Geometry check sheet. Reference: the model listing, model coordinates, mm. Coordinates: 2 decimals unless noted, no trailing zeros. Loops run counter-clockwise (first coordinate to the right, second up) from the corner with the lowest first, then second, coordinate; pieces in that order, holes last.
from build123d import *

# Parameters (mm, degrees)
SKETCH_1_R      = 6
SKETCH_1_R_2    = 3.3
EXTRUDE_1_DEPTH = 5


with BuildPart() as part:
    # 스케치1 → 보스-돌출1 (new body)
    with BuildSketch(Plane(origin=(0, 0, 0), x_dir=(1, 0, 0), z_dir=(0, 1, 0))):
        Circle(SKETCH_1_R)
        Circle(SKETCH_1_R_2, mode=Mode.SUBTRACT)
        with BuildLine():
            Line((-5.795554958, -1.552914271), (-1.448888739, -17.774893441))
            ThreePointArc((-1.448888739, -17.774893441), (0, -18.886664873), (1.448888739, -17.774893441))
            Line((1.448888739, -17.774893441), (5.795554958, -1.552914271))
            ThreePointArc((5.795554958, -1.552914271), (0, -6), (-5.795554958, -1.552914271))
        make_face()
    extrude(amount=EXTRUDE_1_DEPTH)


solid = part.part
1) Section check D-D on x = -4.25. Record the cut outline in (y, z).
Data:
outline: (0, -4.24) - (5, -4.24) - (5, 7.32) - (0, 7.32) - close
2) Mould release check, pull along Z, two halves, no side actions. Record for faces 1 (the flat face through (-3.653, 2.465, 9.55)), 2 (the flat face through (0, 0, 6)), 3 (the cylindrical face through (0, 2, -6)), 4 (the cylindrical face through (-2.43, 2.46, -2.23)): +Z half, -Z half, draft (parallel to the pull), parting line (faces both ways), or undercut.
Data:
face 1: +Z half
face 2: draft
face 3: parting line
face 4: undercut
3) Depth check by flat-ended pin: pin 1 (1.5 mm diameter, centred on y = 2.5, z = 11.5, fed in from +X); pin 2 (1 mm diameter, centred on y = 2, z = 14.5, fed in from +X); pin 3 (2 mm diameter, centred on y = 3, z = 3, fed in from +X); pin 4 (3 mm diameter, centred on x = 2.5, z = 15, fed in from -Y). Enter the tip coordinate at first touch or a pass-through.
Data:
pin 1: stops at x = 3.33
pin 2: stops at x = 2.46
pin 3: stops at x = 5.68
pin 4: stops at y = 0
4) Section check C-C on y = 3.2. Record the cut outline in (x, z), and give its area (3 significant figures).
Data:
outline: (-5.8, 1.55) arc R6 ccw (long way) to (5.8, 1.55) - (1.45, 17.77) arc R1.5 ccw to (-1.45, 17.77) - close; hole circle Ø6.6 at (0, 0)
area: 161 mm2
5) Section check A-A on z = 0. Record the cut outline in (x, y), and give its area (3 significant figures).
Data:
outline: (-6, 0) - (-3.3, 0) - (-3.3, 5) - (-6, 5) - close; (3.3, 0) - (6, 0) - (6, 5) - (3.3, 5) - close
area: 27.0 mm2
6) Material ranges on probe 1 along X at (y, z) = (3.4, 0); probe 2 along X at (y, z) = (3.7, 2); probe 3 along Z at (x, y) = (-1, 3.65), recorded low to high.
Data:
probe 1: x = -6 to -3.3, 3.3 to 6
probe 2: x = -5.68 to -2.62, 2.62 to 5.68
probe 3: z = -5.92 to -3.14, 3.14 to 18.5
7) Section check B-B on x = 0. Record the cut outline in (y, z), and give its area (3 significant figures).
Data:
outline: (0, -6) - (5, -6) - (5, -3.3) - (0, -3.3) - close; (0, 3.3) - (5, 3.3) - (5, 18.89) - (0, 18.89) - close
area: 91.4 mm2
